Geometry: final body of the model. Coordinates: model frame, mm. Round coordinates to 2 decimals unless told otherwise and drop trailing zeros. Loops run counter-clockwise (first coordinate to the right, second up) from the corner with the lowest first, then second, coordinate; pieces in that order, holes last. Notation, with made-up numbers: (-25, -25) - (-6, -25) arc R12 ccw to (-6, -17) - close; hole circle Ø3 at (63.25, 61). An arc over 180 degrees is marked (long way). Answer as CSV lines item,"result".
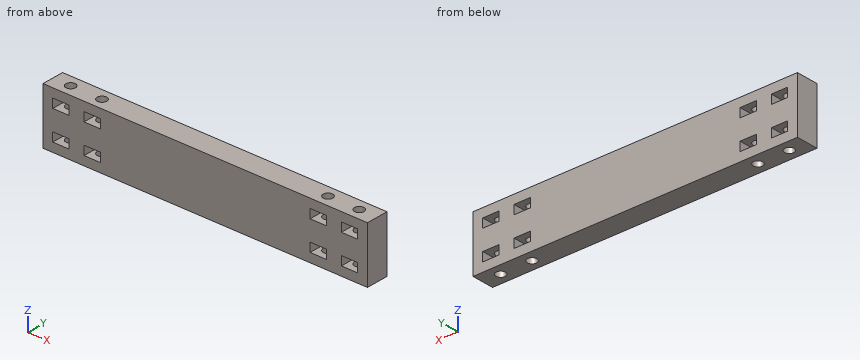
from build123d import *

# Parameters (mm, degrees)
SKETCH1_W           = 145
SKETCH1_H           = 25
BOSS_EXTRUDE1_DEPTH = 10
SKETCH2_R           = 2.15
CUT_EXTRUDE1_DEPTH  = 148.478812038
CUT_EXTRUDE2_REACH  = 149.479
SKETCH3_W           = 7.3
SKETCH3_H           = 4


with BuildPart() as part:
    # Sketch1 → Boss-Extrude1 (new body)
    with BuildSketch(Plane(origin=(0, 0, 0), x_dir=(1, 0, 0), z_dir=(0, 1, 0))):
        with Locations((72.5, 12.5)):
            Rectangle(SKETCH1_W, SKETCH1_H)
    extrude(amount=BOSS_EXTRUDE1_DEPTH)

    # Sketch2 → Cut-Extrude1 (cut, through all)
    with BuildSketch(Plane.XY):
        with Locations((22, 5)):
            Circle(SKETCH2_R)
        with Locations((8, 5)):
            Circle(SKETCH2_R)
        with Locations(Location((123, 5, 0), (0, 0, 180))):
            Circle(SKETCH2_R)
        with Locations(Location((137, 5, 0), (0, 0, 180))):
            Circle(SKETCH2_R)
    extrude(amount=-CUT_EXTRUDE1_DEPTH, mode=Mode.SUBTRACT)

    # Sketch3 → Cut-Extrude2 (cut, up to next)
    with BuildSketch(Plane(origin=(0, 10, 0), x_dir=(1, 0, 0), z_dir=(0, 1, 0)), mode=Mode.PRIVATE) as cut_extrude2_sk1:
        with Locations((137, 19)):
            Rectangle(SKETCH3_W, SKETCH3_H)
    cut_extrude2_tool1 = extrude(cut_extrude2_sk1.sketch, amount=-CUT_EXTRUDE2_REACH, mode=Mode.PRIVATE) & part.part
    # Sketch3 → Cut-Extrude2 (cut, up to next)
    with BuildSketch(Plane(origin=(0, 10, 0), x_dir=(1, 0, 0), z_dir=(0, 1, 0)), mode=Mode.PRIVATE) as cut_extrude2_sk2:
        with Locations((137, 6)):
            Rectangle(SKETCH3_W, SKETCH3_H)
    cut_extrude2_tool2 = extrude(cut_extrude2_sk2.sketch, amount=-CUT_EXTRUDE2_REACH, mode=Mode.PRIVATE) & part.part
    # Sketch3 → Cut-Extrude2 (cut, up to next)
    with BuildSketch(Plane(origin=(0, 10, 0), x_dir=(1, 0, 0), z_dir=(0, 1, 0)), mode=Mode.PRIVATE) as cut_extrude2_sk3:
        with Locations((123, 6)):
            Rectangle(SKETCH3_W, SKETCH3_H)
    cut_extrude2_tool3 = extrude(cut_extrude2_sk3.sketch, amount=-CUT_EXTRUDE2_REACH, mode=Mode.PRIVATE) & part.part
    # Sketch3 → Cut-Extrude2 (cut, up to next)
    with BuildSketch(Plane(origin=(0, 10, 0), x_dir=(1, 0, 0), z_dir=(0, 1, 0)), mode=Mode.PRIVATE) as cut_extrude2_sk4:
        with Locations((123, 19)):
            Rectangle(SKETCH3_W, SKETCH3_H)
    cut_extrude2_tool4 = extrude(cut_extrude2_sk4.sketch, amount=-CUT_EXTRUDE2_REACH, mode=Mode.PRIVATE) & part.part
    # Sketch3 → Cut-Extrude2 (cut, up to next)
    with BuildSketch(Plane(origin=(0, 10, 0), x_dir=(1, 0, 0), z_dir=(0, 1, 0)), mode=Mode.PRIVATE) as cut_extrude2_sk5:
        with Locations((22, 19)):
            Rectangle(SKETCH3_W, SKETCH3_H)
    cut_extrude2_tool5 = extrude(cut_extrude2_sk5.sketch, amount=-CUT_EXTRUDE2_REACH, mode=Mode.PRIVATE) & part.part
    # Sketch3 → Cut-Extrude2 (cut, up to next)
    with BuildSketch(Plane(origin=(0, 10, 0), x_dir=(1, 0, 0), z_dir=(0, 1, 0)), mode=Mode.PRIVATE) as cut_extrude2_sk6:
        with Locations((22, 6)):
            Rectangle(SKETCH3_W, SKETCH3_H)
    cut_extrude2_tool6 = extrude(cut_extrude2_sk6.sketch, amount=-CUT_EXTRUDE2_REACH, mode=Mode.PRIVATE) & part.part
    # Sketch3 → Cut-Extrude2 (cut, up to next)
    with BuildSketch(Plane(origin=(0, 10, 0), x_dir=(1, 0, 0), z_dir=(0, 1, 0)), mode=Mode.PRIVATE) as cut_extrude2_sk7:
        with Locations((8, 19)):
            Rectangle(SKETCH3_W, SKETCH3_H)
    cut_extrude2_tool7 = extrude(cut_extrude2_sk7.sketch, amount=-CUT_EXTRUDE2_REACH, mode=Mode.PRIVATE) & part.part
    # Sketch3 → Cut-Extrude2 (cut, up to next)
    with BuildSketch(Plane(origin=(0, 10, 0), x_dir=(1, 0, 0), z_dir=(0, 1, 0)), mode=Mode.PRIVATE) as cut_extrude2_sk8:
        with Locations((8, 6)):
            Rectangle(SKETCH3_W, SKETCH3_H)
    cut_extrude2_tool8 = extrude(cut_extrude2_sk8.sketch, amount=-CUT_EXTRUDE2_REACH, mode=Mode.PRIVATE) & part.part
    add(cut_extrude2_tool1.solids().sort_by_distance((137, 10, -19))[0], mode=Mode.SUBTRACT)
    add(cut_extrude2_tool2.solids().sort_by_distance((137, 10, -6))[0], mode=Mode.SUBTRACT)
    add(cut_extrude2_tool3.solids().sort_by_distance((123, 10, -6))[0], mode=Mode.SUBTRACT)
    add(cut_extrude2_tool4.solids().sort_by_distance((123, 10, -19))[0], mode=Mode.SUBTRACT)
    add(cut_extrude2_tool5.solids().sort_by_distance((22, 10, -19))[0], mode=Mode.SUBTRACT)
    add(cut_extrude2_tool6.solids().sort_by_distance((22, 10, -6))[0], mode=Mode.SUBTRACT)
    add(cut_extrude2_tool7.solids().sort_by_distance((8, 10, -19))[0], mode=Mode.SUBTRACT)
    add(cut_extrude2_tool8.solids().sort_by_distance((8, 10, -6))[0], mode=Mode.SUBTRACT)


solid = part.part
(1) Section B-B (z = -18.25). Output: boundary loops of the cut face in (x, y), and give its area (3 significant figures).
Findings below:
outline,"(0, 0) - (4.35, 0) - (4.35, 10) - (0, 10) - close; (11.65, 0) - (18.35, 0) - (18.35, 10) - (11.65, 10) - close; (25.65, 0) - (119.35, 0) - (119.35, 10) - (25.65, 10) - close; (126.65, 0) - (133.35, 0) - (133.35, 10) - (126.65, 10) - close; (140.65, 0) - (145, 0) - (145, 10) - (140.65, 10) - close"
area,"1,160 mm2"
(2) Material intervals for line 1 along X through (y, z) = (9.25, -19.25); line 2 along Y through (x, z) = (137, -0.8), sorted ascending.
Findings below:
line 1,"0 to 4.35, 11.65 to 18.35, 25.65 to 119.35, 126.65 to 133.35, 140.65 to 145"
line 2,"0 to 2.85, 7.15 to 10"
(3) Section A-A (x = 22). Output: boundary loops of the cut face in (y, z), and give its area (3 significant figures).
Findings below:
outline,"(0, -25) - (2.85, -25) - (2.85, -21) - (0, -21) - close; (0, -17) - (2.85, -17) - (2.85, -8) - (0, -8) - close; (0, -4) - (2.85, -4) - (2.85, 0) - (0, 0) - close; (7.15, -25) - (10, -25) - (10, -21) - (7.15, -21) - close; (7.15, -17) - (10, -17) - (10, -8) - (7.15, -8) - close; (7.15, -4) - (10, -4) - (10, 0) - (7.15, 0) - close"
area,"96.9 mm2"
(4) Section C-C (z = -11.25). Output: boundary loops of the cut face in (x, y), and give its area (3 significant figures).
Findings below:
outline,"(0, 0) - (145, 0) - (145, 10) - (0, 10) - close; hole circle Ø4.3 at (8, 5); hole circle Ø4.3 at (22, 5); hole circle Ø4.3 at (123, 5); hole circle Ø4.3 at (137, 5)"
area,"1,390 mm2"
